For this review, take the finished solid that the model builds, in its own axes (mm). A direction names the side the tool comes from. Coordinates: 2 decimals unless noted, no trailing zeros. Write each loop counter-clockwise with the first axis right and the second up, starting at its lowest first coordinate (ties: lowest second). Pieces come first, ordered by that corner, then holes.
1) We need section B-B on z = -2.25. Write out the cut boundary in (x, y).
2) Mouldability with a two-part tool opening along Y and no side actions: class faces 1 (the face through (12, 0, -7)), 2 (the face through (12, -6, -3)), 3 (the face through (0, 8, 1)), 4 (the face through (-20.2, 0.05, 1.01)) as pulls with the +Y half, pulls with the -Y half, needs draft (parallel to the pull), parting line crosses it, or undercut.
3) We need section D-D on x = -11.5. Write out the cut boundary in (y, z), then the cut area to 3 significant figures.
4) For faces 5 (the face through (-12, 6, -3)), 6 (the face through (-15, 0, -3)), 7 (the face through (0, -5, 8)), 8 (the face through (-12, -6, -3)), 9 (the face through (-7, 0, 8)), list the 3-axis set-ups (+Z, -Z, +X, -X, +Y, -Y) from which the entire face can be reached by the end or side of a thin tool; tool diameter is ignored.
5) We need section A-A on y = 0. Write out the cut boundary in (x, z), then the cut area to 3 significant figures.
6) Insertion check: P1, Ø1, axis at y = -1, z = -3.5, coming from the -X side; P2, Ø3, axis at x = 12.5, z = -4.5, coming from the -Y side; P3, Ø5, axis at y = -1, z = 10, coming from the +X side. Each pin has a flat end and moves straight along its axis. Give the tip position at first contact, or say it passes through.
7) To check wall thickness, follow line 1 along Y through (x, z) = (-19, 0.9); line 2 along X through (y, z) = (-0.5, 1.75); line 3 along X through (y, z) = (5.5, -1.75). State the ranges of each line that lie inside material, in increasing order.
8) We need section C-C on x = 19. Write out the cut boundary in (y, z).
from build123d import *

# Parameters (mm, degrees)
SKETCH_1_W          = 45
SKETCH_1_H          = 16
EXTRUDE_1_DEPTH     = 2
SKETCH_2_R          = 1.2
CUT_EXTRUDE_1_DEPTH = 2
SKETCH_3_W          = 14
SKETCH_3_H          = 10
EXTRUDE_2_DEPTH     = 13
SKETCH_4_W          = 6
SKETCH_4_H          = 12
EXTRUDE_3_DEPTH     = 9


with BuildPart() as part:
    # ｽｹｯﾁ1 → ﾎﾞｽ - 押し出し1 (new body)
    with BuildSketch(Plane.XY):
        Rectangle(SKETCH_1_W, SKETCH_1_H)
    extrude(amount=EXTRUDE_1_DEPTH)

    # ｽｹｯﾁ2 → ｶｯﾄ - 押し出し1 (cut)
    with BuildSketch(Plane.XY.offset(2)):
        with Locations((-19, 0)):
            Circle(SKETCH_2_R)
        with Locations((19, 0)):
            Circle(SKETCH_2_R)
    extrude(amount=-CUT_EXTRUDE_1_DEPTH, mode=Mode.SUBTRACT)

    # ｽｹｯﾁ3 → ﾎﾞｽ - 押し出し2 (add)
    with BuildSketch(Plane.XY.offset(2)):
        Rectangle(SKETCH_3_W, SKETCH_3_H)
    extrude(amount=EXTRUDE_2_DEPTH)

    # ｽｹｯﾁ4 → ﾎﾞｽ - 押し出し3 (add)
    with BuildSketch(Plane.XY.offset(2)):
        with Locations((-12, 0)):
            Rectangle(SKETCH_4_W, SKETCH_4_H)
        with Locations((12, 0)):
            Rectangle(SKETCH_4_W, SKETCH_4_H)
    extrude(amount=-EXTRUDE_3_DEPTH)


solid = part.part
Result:
1. outline: (-15, -6) - (-9, -6) - (-9, 6) - (-15, 6) - close; (9, -6) - (15, -6) - (15, 6) - (9, 6) - close
2. face 1: needs draft
2. face 2: pulls with the -Y half
2. face 3: pulls with the +Y half
2. face 4: undercut
3. outline: (-8, 0) - (-6, 0) - (-6, -7) - (6, -7) - (6, 0) - (8, 0) - (8, 2) - (-8, 2) - close
3. area: 116 mm2
4. face 5: -Z, +X, -X, +Y
4. face 6: -Z, -X, +Y, -Y
4. face 7: +Z, +X, -X, -Y
4. face 8: -Z, +X, -X, -Y
4. face 9: +Z, -X, +Y, -Y
5. outline: (-22.5, 0) - (-20.2, 0) - (-20.2, 2) - (-22.5, 2) - close; (-17.8, 0) - (-15, 0) - (-15, -7) - (-9, -7) - (-9, 0) - (9, 0) - (9, -7) - (15, -7) - (15, 0) - (17.8, 0) - (17.8, 2) - (7, 2) - (7, 15) - (-7, 15) - (-7, 2) - (-17.8, 2) - close; (20.2, 0) - (22.5, 0) - (22.5, 2) - (20.2, 2) - close
5. area: 346 mm2
6. P1: stops at x = -15
6. P2: stops at y = -6
6. P3: stops at x = 7
7. line 1: y = -8 to -1.2, 1.2 to 8
7. line 2: x = -22.5 to -20.09, -17.91 to 17.91, 20.09 to 22.5
7. line 3: x = -15 to -9, 9 to 15
8. outline: (-8, 0) - (-1.2, 0) - (-1.2, 2) - (-8, 2) - close; (1.2, 0) - (8, 0) - (8, 2) - (1.2, 2) - close
